Input: dimensioned drawing with shaded views. Units: mm. Origin: part minimum x, y, z. A direction names the side the tool comes from. Round coordinates to 2 decimals unless told otherwise and drop trailing zeros. Loops run counter-clockwise (first coordinate to the right, second up) from the corner with the lowest first, then second, coordinate; pieces in that order, holes last.
Item 1: Access query for the marked faces 1 and 2. Directions: +Z, -Z, +X, -X, +Y, -Y. A direction counts if a zero-diameter tool reaches every point of the face in a straight line with its end or side. Return the directions, or none.
Item 2: Section query D-D on x = 16. Return loops of the section in (y, z), then the cut area to 3 significant figures.
Item 3: Section query A-A on x = 43.5. Return loops of the section in (y, z), then the cut area to 3 significant figures.
Item 4: Ray query, L1, parallel to Z at x = 45.8, y = 5.5; L2, parallel to Y at x = 43, z = 36 (1 decimal). Return the intervals inside material, ascending.
Item 5: Section query B-B on y = 21. Return loops of the section in (x, z), then the cut area to 3 significant figures.
Item 6: First-contact query: P1, Ø12.5, axis at y = 26.5, z = 14, coming from the +X side; P2, Ø1.5, axis at y = 37, z = 37, coming from the +X side; P3, Ø0.8, axis at x = 5.5, z = 42.5, coming from the -Y side. Flat tips, straight axial feed; report the tip coordinate or a pass-through.
Item 7: Section query C-C on z = 26. Return loops of the section in (x, y).
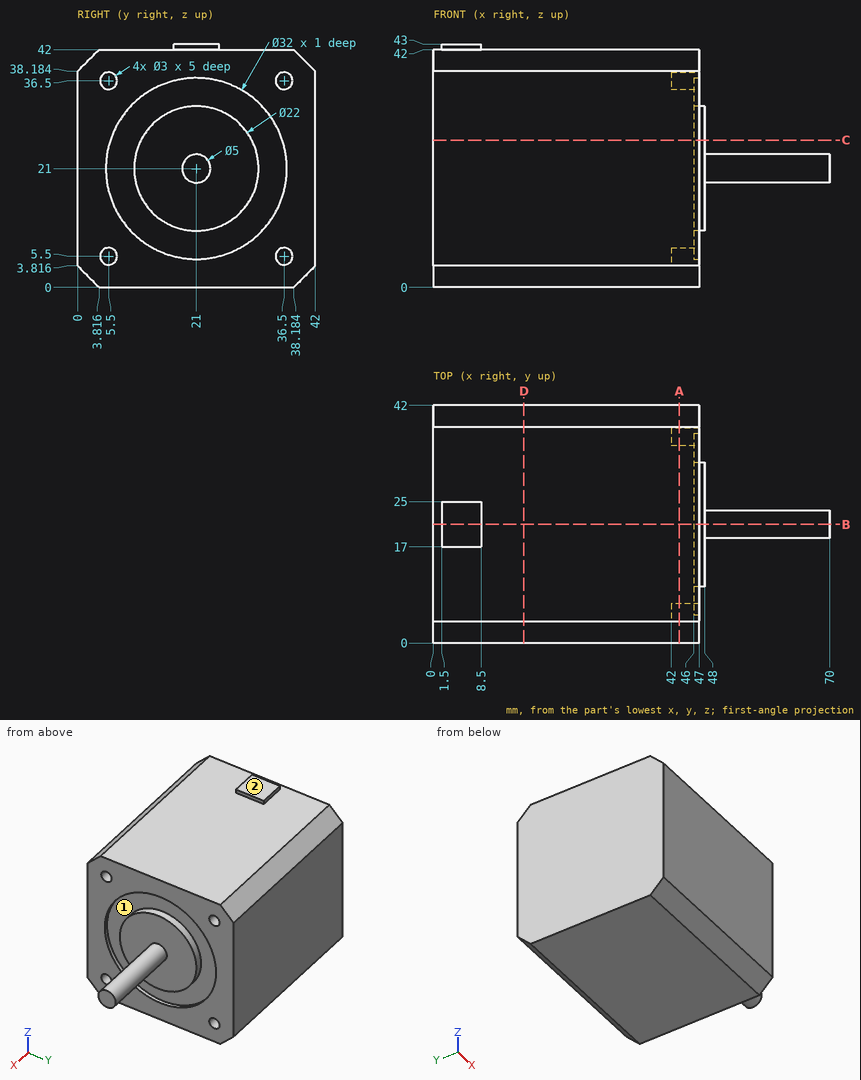
Data:
1. face 1: +X
1. face 2: +Z, +X, -X, +Y, -Y
2. outline: (0, 3.82) - (3.82, 0) - (38.18, 0) - (42, 3.82) - (42, 38.18) - (38.18, 42) - (3.82, 42) - (0, 38.18) - close
2. area: 1,730 mm2
3. outline: (0, 3.82) - (3.82, 0) - (38.18, 0) - (42, 3.82) - (42, 38.18) - (38.18, 42) - (3.82, 42) - (0, 38.18) - close; hole circle Ø3 at (5.5, 5.5); hole circle Ø3 at (5.5, 36.5); hole circle Ø3 at (36.5, 5.5); hole circle Ø3 at (36.5, 36.5)
3. area: 1,710 mm2
4. L1: z = 0 to 4, 7 to 35, 38 to 42
4. L2: y = 0 to 4.1, 6.9 to 35.1, 37.9 to 42
5. outline: (0, 0) - (47, 0) - (47, 5) - (46, 5) - (46, 10) - (48, 10) - (48, 18.5) - (70, 18.5) - (70, 23.5) - (48, 23.5) - (48, 32) - (46, 32) - (46, 37) - (47, 37) - (47, 42) - (8.5, 42) - (8.5, 43) - (1.5, 43) - (1.5, 42) - (0, 42) - close
5. area: 2,100 mm2
6. P1: stops at x = 48
6. P2: stops at x = 42
6. P3: stops at y = 17
7. outline: (0, 0) - (47, 0) - (47, 5.8) - (46, 5.8) - (46, 11.2) - (48, 11.2) - (48, 30.8) - (46, 30.8) - (46, 36.2) - (47, 36.2) - (47, 42) - (0, 42) - close
